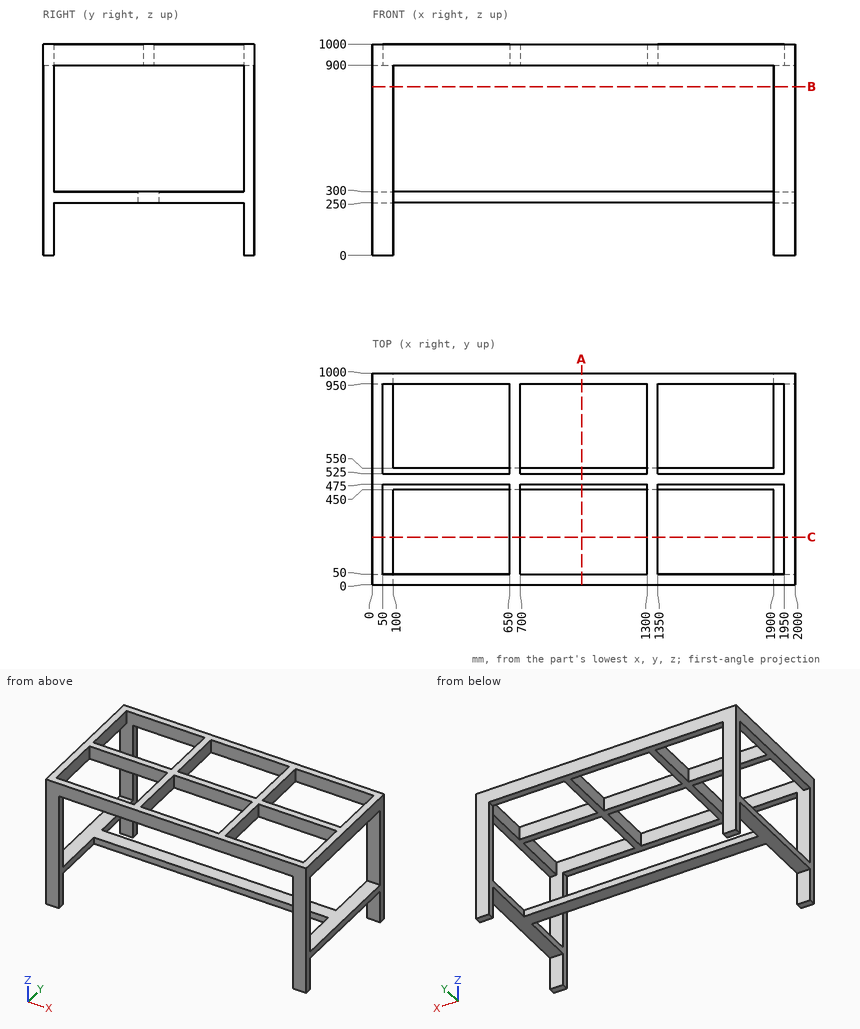
Geometry: see drawing. Coordinates: mm, zero at the bounding-box minimum. Give positions to 0.01 mm unless a question says otherwise; leave off trailing zeros. Write each loop counter-clockwise with the first axis right and the second up, starting at its lowest first coordinate (ties: lowest second). Pieces come first, ordered by that corner, then holes. Notation, with made-up numbers: (14.25, 20) -> (67.25, 20) arc R24 cw to (67.25, 37) -> close; hole circle Ø1 at (37.25, 58.5). An arc over 180 degrees is marked (long way). Use one line per item in the form item = value. Start each with the question number.
1) Section query B-B on z = 798.5. Return the cut outline in (x, y).
2) Pin query (flat end, axial travel): pin 1 (3 mm diameter, centred on x = 1640.5, y = 458.5, fed in from -Z); pin 2 (25 mm diameter, centred on x = 1288, z = 270.5, fed in from +Y). Return the tip coordinate at first contact, or that it passes through.
3) Section query A-A on x = 990.5. Return the cut outline in (y, z), then the cut area to 3 significant figures.
4) Section query C-C on y = 225. Return the cut outline in (x, z).
5) Ray query, probe 1 along X at (y, z) = (356, 948.5); probe 2 along Y at (x, z) = (1765, 903); probe 3 along X at (y, z) = (900, 295.5). Return the intervals inside material, ascending. Write a range as from..to.
Outcome:
q1.outline = (0, 0) -> (100, 0) -> (100, 50) -> (0, 50) -> close; (0, 950) -> (100, 950) -> (100, 1000) -> (0, 1000) -> close; (1900, 0) -> (2000, 0) -> (2000, 50) -> (1900, 50) -> close; (1900, 950) -> (2000, 950) -> (2000, 1000) -> (1900, 1000) -> close
q2.pin_1 = 250
q2.pin_2 = 550
q3.outline = (0, 900) -> (50, 900) -> (50, 1000) -> (0, 1000) -> close; (450, 250) -> (550, 250) -> (550, 300) -> (450, 300) -> close; (475, 900) -> (525, 900) -> (525, 1000) -> (475, 1000) -> close; (950, 900) -> (1000, 900) -> (1000, 1000) -> (950, 1000) -> close
q3.area = 20,000 mm^2
q4.outline = (0, 250) -> (100, 250) -> (100, 300) -> (0, 300) -> close; (0, 900) -> (50, 900) -> (50, 1000) -> (0, 1000) -> close; (650, 900) -> (700, 900) -> (700, 1000) -> (650, 1000) -> close; (1300, 900) -> (1350, 900) -> (1350, 1000) -> (1300, 1000) -> close; (1900, 250) -> (2000, 250) -> (2000, 300) -> (1900, 300) -> close; (1950, 900) -> (2000, 900) -> (2000, 1000) -> (1950, 1000) -> close
q5.probe_1 = 0..50, 650..700, 1300..1350, 1950..2000
q5.probe_2 = 0..50, 475..525, 950..1000
q5.probe_3 = 0..100, 1900..2000
